Check sheet for the drawn part. Datum: minimum x, y, z corner. Units: mm. A direction names the side the tool comes from. Coordinates: 2 decimals unless noted, no trailing zeros. Order: outer loops, then holes, each group sorted by start corner. A loop starts at its lowest first (then second) coordinate and runs counter-clockwise, first axis right, second up. Notation, with made-up numbers: (38, 40.5) -> (81, 40.5) arc R22 cw to (81, 68.5) -> close; hole circle Ø11 at (-30.5, -24.5). An arc over 180 degrees is marked (long way). Answer as CSV lines item,"result".
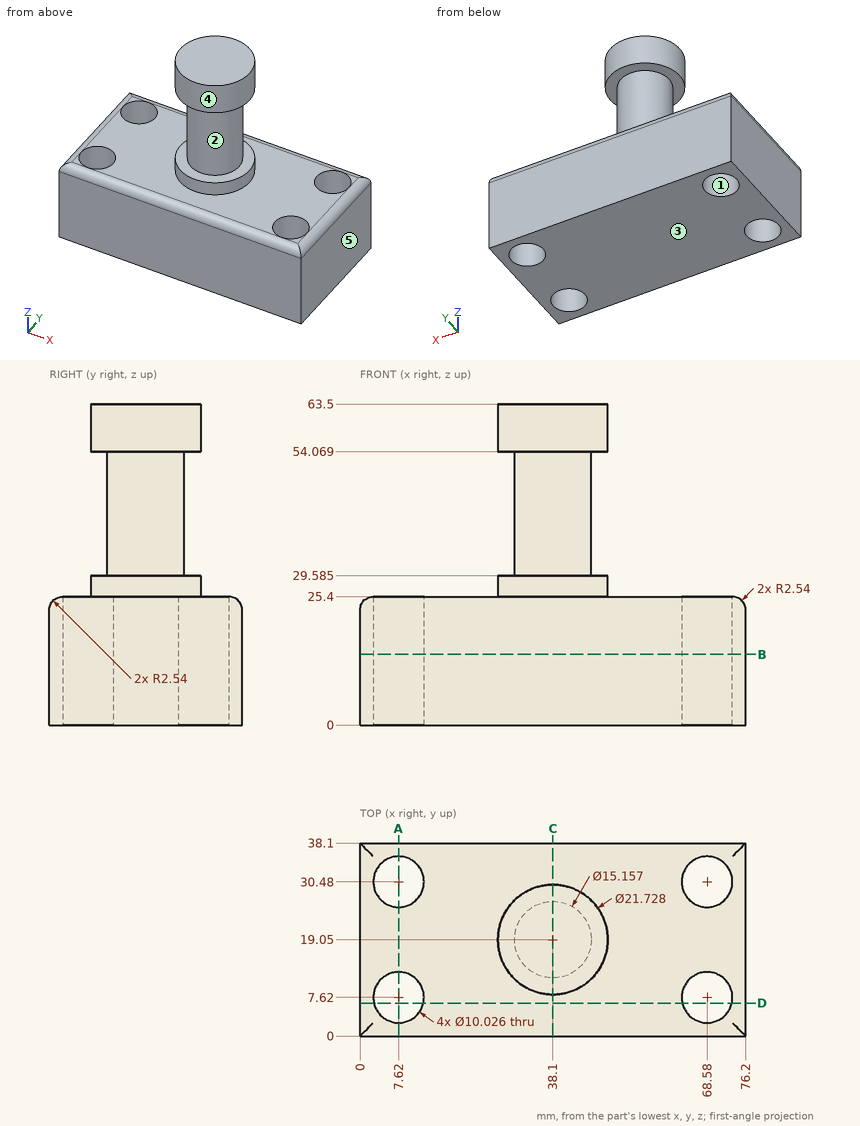
Item 1: Section check A-A, the plane x = 7.62. Record the boundary of the cut face in (y, z).
Answer list:
outline,"(0, 0) -> (2.61, 0) -> (2.61, 25.4) -> (2.54, 25.4) arc R2.54 ccw to (0, 22.86) -> close; (12.63, 0) -> (25.47, 0) -> (25.47, 25.4) -> (12.63, 25.4) -> close; (35.49, 0) -> (38.1, 0) -> (38.1, 22.86) arc R2.54 ccw to (35.56, 25.4) -> (35.49, 25.4) -> close"
Item 2: Section check D-D, the plane y = 6.5. Record the boundary of the cut face in (x, z), plus the area to 3 significant figures.
Answer list:
outline,"(0, 0) -> (2.73, 0) -> (2.73, 25.4) -> (2.54, 25.4) arc R2.54 ccw to (0, 22.86) -> close; (12.51, 0) -> (63.69, 0) -> (63.69, 25.4) -> (12.51, 25.4) -> close; (73.47, 0) -> (76.2, 0) -> (76.2, 22.86) arc R2.54 ccw to (73.66, 25.4) -> (73.47, 25.4) -> close"
area,"1,440 mm2"
Item 3: Depth check by flat-ended pin: pin 1 Ø12 at (y, z) = (13.5, 38.5) entering from +X; pin 2 Ø3 at (x, z) = (43, 26.5) entering from -Y; pin 3 Ø6 at (x, z) = (39.5, 29) entering from -Y. Enter the tip coordinate at first touch or a pass-through.
Answer list:
pin 1,"x = 45.68"
pin 2,"y = 1.17"
pin 3,"y = 8.19"
Item 4: Tool access check on the marked faces 4 and 5. Record the directions out of +Z, -Z, +X, -X, +Y, -Y that give a thin tool (end or side, any length) a straight path to the whole face; none if there is none.
Answer list:
face 4,"+Z"
face 5,"+Z, -Z, +X, +Y, -Y"
Item 5: Section check B-B, the plane z = 14. Record the boundary of the cut face in (x, y), plus the area to 3 significant figures.
Answer list:
outline,"(0, 0) -> (76.2, 0) -> (76.2, 38.1) -> (0, 38.1) -> close; hole circle Ø10.03 at (7.62, 7.62); hole circle Ø10.03 at (7.62, 30.48); hole circle Ø10.03 at (68.58, 7.62); hole circle Ø10.03 at (68.58, 30.48)"
area,"2,590 mm2"
Item 6: Section check C-C, the plane x = 38.1. Record the boundary of the cut face in (y, z) (1 decimal).
Answer list:
outline,"(0, 0) -> (38.1, 0) -> (38.1, 22.9) arc R2.5 ccw to (35.6, 25.4) -> (29.9, 25.4) -> (29.9, 29.6) -> (26.6, 29.6) -> (26.6, 54.1) -> (29.9, 54.1) -> (29.9, 63.5) -> (8.2, 63.5) -> (8.2, 54.1) -> (11.5, 54.1) -> (11.5, 29.6) -> (8.2, 29.6) -> (8.2, 25.4) -> (2.5, 25.4) arc R2.5 ccw to (0, 22.9) -> close"
Item 7: Thickness scan on line 1 (Y direction, x = 68.58, z = 19); line 2 (Z direction, x = 30.5, y = 22) (1 decimal); line 3 (Z direction, x = 42, y = 32.5). Record the ranges inside material, lowest first.
Answer list:
line 1,"0 to 2.61, 12.63 to 25.47, 35.49 to 38.1"
line 2,"0 to 29.6, 54.1 to 63.5"
line 3,"0 to 25.4"
Item 8: Release check for a two-part mould opening along Z. For the marked faces 1, 2 and 3 record: +Z half, -Z half, draft (parallel to the pull), parting line (faces both ways), or undercut.
Answer list:
face 1,"draft"
face 2,"undercut"
face 3,"-Z half"
